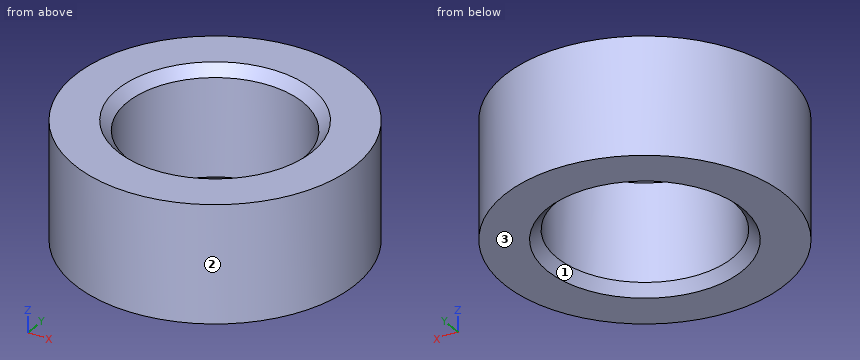
```python
from build123d import *

# Parameters (mm, degrees)
F0_R     = 7.2
F1_DEPTH = 6
F2_R     = 4.5
F3_DEPTH = 25
F4_SIZE2 = 0.5
F4_SIZE  = 0.5


with BuildPart() as f1:
    # F0 (on Top) → F1 (new body)
    with BuildSketch(Plane.XY):
        Circle(F0_R)
    extrude(amount=F1_DEPTH)

    # F2 (on face) → F3 (cut)
    with BuildSketch(Plane.XY.offset(6)):
        Circle(F2_R)
    extrude(amount=-F3_DEPTH, mode=Mode.SUBTRACT)

    # F4
    f4_edges = [f1.edges().sort_by_distance(p)[0] for p in [
        (-4.5, 0, 6),
        (-4.5, 0, 0),
    ]]
    chamfer(f4_edges, length=F4_SIZE, length2=F4_SIZE2)


solid = f1.part
```
Geometry: final body of the model. Coordinates: model frame, mm. Face numbers are marked on the shaded views. Coordinates: 2 decimals unless noted, no trailing zeros. Order: outer loops, then holes, each group sorted by start corner. A loop starts at its lowest first (then second) coordinate and runs counter-clockwise, first axis right, second up.
Item 1: Material intervals for line 1 along Y through (x, z) = (0, 4); line 2 along X through (y, z) = (2.5, 3.05); line 3 along X through (y, z) = (-0.5, 5.3), sorted ascending.
Answer:
line 1: y = -7.2 to -4.5, 4.5 to 7.2
line 2: x = -6.75 to -3.74, 3.74 to 6.75
line 3: x = -7.18 to -4.47, 4.47 to 7.18
Item 2: Section query A-A (y = 0). Output: boundary loops of the cut face in (x, z).
Answer:
outline: (-7.2, 0) - (-5, 0) - (-4.5, 0.5) - (-4.5, 5.5) - (-5, 6) - (-7.2, 6) - close; (4.5, 0.5) - (5, 0) - (7.2, 0) - (7.2, 6) - (5, 6) - (4.5, 5.5) - close
Item 3: Draft query along Y for the marked faces 1, 2 and 3. Return one class per face: released by +Y, released by -Y, zero draft, split by the parting line, or undercut.
Answer:
face 1: undercut
face 2: split by the parting line
face 3: zero draft
Item 4: Section query D-D (x = 5.75). Output: boundary loops of the cut face in (y, z), then the cut area to 3 significant figures.
Answer:
outline: (-4.33, 0) - (4.33, 0) - (4.33, 6) - (-4.33, 6) - close
area: 52.0 mm2
Item 5: Section query C-C (z = 4.8). Output: boundary loops of the cut face in (x, y), then the cut area to 3 significant figures.
Answer:
outline: circle Ø14.4 at (0, 0); hole circle Ø9 at (0, 0)
area: 99.2 mm2
Item 6: Contact query for a flat-ended pin moving along its axis: P1, Ø3, axis at x = 5.5, z = 3, coming from the +Y side. Output: stop coordinate, or through.
Answer:
P1: stops at y = 5.99
